from build123d import *

# Parameters (mm, degrees)
SKETCH_1_R                      = 21
EXTRUDE_1_DEPTH                 = 1.5
SKETCH_2_R                      = 21
SKETCH_2_R_2                    = 12
EXTRUDE_2_DEPTH                 = 2.2
SKETCH_7_R                      = 1.25
CUT_EXTRUDE_5_DEPTH             = 30.92808046
SKETCH_8_W                      = 14.034551426
SKETCH_8_H                      = 10.5
CUT_EXTRUDE_6_DEPTH             = 30.92808046
SKETCH_9_W                      = 17.42220177
SKETCH_9_H                      = 10.5
CUT_EXTRUDE_7_DEPTH             = 30.92808046
MOVE_BODY_5_ANGLE               = 45
MOVE_BODY_6_ANGLE               = 5
SKETCH_15_R                     = 0.55
SKETCH_15_R_2                   = 0.5
CUT_EXTRUDE_9_DEPTH             = 30.92808046
MOVE_BODY_7_ANGLE               = 49.5
SKETCH_16_R                     = 1.35
CUT_EXTRUDE_10_DEPTH            = 1.5
SKETCH_17_R                     = 2.5
CUT_EXTRUDE_11_DEPTH            = 2.2
SKETCH_23_R                     = 2
CUT_EXTRUDE_17_DEPTH            = 30.92808046
CUT_EXTRUDE_18_DEPTH            = 30.779858965
CUT_EXTRUDE_18_DEPTH_BACK       = 30.779858965
SKETCH_24_R                     = 1.6
CUT_EXTRUDE_25_DEPTH            = 30.92808046
SKETCH_42_R                     = 3
CUT_EXTRUDE_26_DEPTH            = 1
HOLE_WIZARD_3_100_1_D           = 3.048
HOLE_WIZARD_3_100_1_CSINK_D     = 5.0546
HOLE_WIZARD_3_100_1_CSINK_ANGLE = 100
CUT_EXTRUDE_27_DEPTH            = 30.92808046


with BuildPart() as part:
    # 草图1 → 凸台-拉伸1 (new body)
    with BuildSketch(Plane(origin=(0, 0, 0), x_dir=(1, 0, 0), z_dir=(0, 1, 0))):
        with Locations(Location((0, 0, 0), (0, 0, 270))):
            Circle(SKETCH_1_R)
    extrude(amount=EXTRUDE_1_DEPTH)

    # 草图2 → 凸台-拉伸2 (add)
    with BuildSketch(Plane(origin=(0, 1.5, 0), x_dir=(1, 0, 0), z_dir=(0, 1, 0))):
        with Locations(Location((0, 0, 0), (0, 0, 270))):
            Circle(SKETCH_2_R)
        with Locations(Location((0, 0, 0), (0, 0, 270))):
            Circle(SKETCH_2_R_2, mode=Mode.SUBTRACT)
    extrude(amount=EXTRUDE_2_DEPTH)

    # 草图7 → 切除-拉伸5 (cut, through all)
    with BuildSketch(Plane.XZ):
        with Locations(Location((-5.51, 9.05, 0), (0, 0, 270))):
            Circle(SKETCH_7_R)
        with Locations(Location((5.51, 9.05, 0), (0, 0, 270))):
            Circle(SKETCH_7_R)
        with Locations(Location((-5.51, -9.05, 0), (0, 0, 270))):
            Circle(SKETCH_7_R)
        with Locations(Location((5.51, -9.05, 0), (0, 0, 270))):
            Circle(SKETCH_7_R)
    extrude(amount=-CUT_EXTRUDE_5_DEPTH, mode=Mode.SUBTRACT)

    # 草图8 → 切除-拉伸6 (cut, through all)
    with BuildSketch(Plane.XZ):
        Rectangle(SKETCH_8_W, SKETCH_8_H)
    extrude(amount=-CUT_EXTRUDE_6_DEPTH, mode=Mode.SUBTRACT)

    # 草图9 → 切除-拉伸7 (cut, through all)
    with BuildSketch(Plane.XZ):
        with Locations((15.728376598, 0)):
            Rectangle(SKETCH_9_W, SKETCH_9_H)
    extrude(amount=-CUT_EXTRUDE_7_DEPTH, mode=Mode.SUBTRACT)


with BuildPart() as part_1:
    # Move Body 5: moved
    add(part.part.rotate(Axis((0, 0, 0), (0, 1, 0)), MOVE_BODY_5_ANGLE))


with BuildPart() as part_2:
    # Move Body 6: moved
    add(part_1.part.rotate(Axis((0, 0, 0), (0, 1, 0)), MOVE_BODY_6_ANGLE))

    # 草图15 → 切除-拉伸9 (cut, through all)
    with BuildSketch(Plane.XZ):
        with Locations(Location((-10.9, 10.9, 0), (0, 0, 270))):
            Circle(SKETCH_15_R)
        with Locations(Location((10.9, 10.9, 0), (0, 0, 270))):
            Circle(SKETCH_15_R_2)
        with Locations(Location((-10.9, -10.9, 0), (0, 0, 270))):
            Circle(SKETCH_15_R_2)
    extrude(amount=-CUT_EXTRUDE_9_DEPTH, mode=Mode.SUBTRACT)


with BuildPart() as part_3:
    # Move Body 7: moved
    add(part_2.part.rotate(Axis((0, 0, 0), (0, -1, 0)), MOVE_BODY_7_ANGLE))

    # 草图16 → 切除-拉伸10 (cut)
    with BuildSketch(Plane.XZ):
        with Locations(Location((-5.51, 9.05, 0), (0, 0, 270))):
            Circle(SKETCH_16_R)
        with Locations(Location((5.51, 9.05, 0), (0, 0, 270))):
            Circle(SKETCH_16_R)
        with Locations(Location((-5.51, -9.05, 0), (0, 0, 270))):
            Circle(SKETCH_16_R)
        with Locations(Location((5.51, -9.05, 0), (0, 0, 270))):
            Circle(SKETCH_16_R)
    extrude(amount=-CUT_EXTRUDE_10_DEPTH, mode=Mode.SUBTRACT)

    # 草图17 → 切除-拉伸11 (cut)
    with BuildSketch(Plane(origin=(0, 3.7, 0), x_dir=(1, 0, 0), z_dir=(0, 1, 0))):
        with Locations((-5.51, 9.05)):
            Circle(SKETCH_17_R)
        with Locations((5.51, 9.05)):
            Circle(SKETCH_17_R)
        with Locations((-5.51, -9.05)):
            Circle(SKETCH_17_R)
        with Locations((5.51, -9.05)):
            Circle(SKETCH_17_R)
    extrude(amount=-CUT_EXTRUDE_11_DEPTH, mode=Mode.SUBTRACT)

    # 草图23 → 切除-拉伸17 (cut, through all)
    with BuildSketch(Plane(origin=(0, 3.7, 0), x_dir=(1, 0, 0), z_dir=(0, 1, 0))):
        with Locations(Location((0, 16, 0), (0, 0, 270))):
            Circle(SKETCH_23_R)
        with Locations(Location((-16, 0, 0), (0, 0, 270))):
            Circle(SKETCH_23_R)
        with Locations(Location((0, -16, 0), (0, 0, 270))):
            Circle(SKETCH_23_R)
    extrude(amount=-CUT_EXTRUDE_17_DEPTH, mode=Mode.SUBTRACT)

    # 草图24 → 切除-拉伸18 (cut, two sides: drawn at the far end of the back side and taken through both)
    with BuildSketch(Plane(origin=(0, 1.5, 0), x_dir=(1, 0, 0), z_dir=(0, 1, 0)).offset(-CUT_EXTRUDE_18_DEPTH_BACK)):
        with Locations(Location((-5.51, 9.05, 0), (0, 0, 270))):
            Circle(SKETCH_24_R)
        with Locations(Location((5.51, 9.05, 0), (0, 0, 270))):
            Circle(SKETCH_24_R)
        with Locations(Location((-5.51, -9.05, 0), (0, 0, 270))):
            Circle(SKETCH_24_R)
        with Locations(Location((5.51, -9.05, 0), (0, 0, 270))):
            Circle(SKETCH_24_R)
    extrude(amount=CUT_EXTRUDE_18_DEPTH + CUT_EXTRUDE_18_DEPTH_BACK, mode=Mode.SUBTRACT)

    # 草图37 → 切除-拉伸25 (cut, through all)
    with BuildSketch(Plane.XZ):
        with BuildLine():
            Line((24.72756624, 20.266700409), (14.622140931, 20.266700409))
            Line((14.622140931, 20.266700409), (14.622140931, 15.072922563))
            ThreePointArc((14.622140931, 15.072922563), (18.200516902, 10.47574267), (20.378202654, 5.072362031))
            Line((20.378202654, 5.072362031), (14.622140931, 5.122594421))
            Line((14.622140931, 5.122594421), (14.622140931, -5.377805402))
            Line((14.622140931, -5.377805402), (20.286574032, -5.427238161))
            ThreePointArc((20.286574032, -5.427238161), (18.108406942, -10.634171243), (14.622140931, -15.072922563))
            Line((14.622140931, -15.072922563), (14.622140931, -20.266073881))
            Line((14.622140931, -20.266073881), (24.72756624, -20.266073881))
            Line((24.72756624, -20.266073881), (24.72756624, 20.266700409))
        make_face()
        with BuildLine():
            ThreePointArc((20.378202654, 5.072362031), (18.200516902, 10.47574267), (14.622140931, 15.072922563))
            Line((14.622140931, 15.072922563), (14.622140931, 5.122594421))
            Line((14.622140931, 5.122594421), (20.378202654, 5.072362031))
        make_face()
        with BuildLine():
            Line((14.622140931, -5.377805402), (14.622140931, -15.072922563))
            ThreePointArc((14.622140931, -15.072922563), (18.108406942, -10.634171243), (20.286574032, -5.427238161))
            Line((20.286574032, -5.427238161), (14.622140931, -5.377805402))
        make_face()
    extrude(amount=-CUT_EXTRUDE_25_DEPTH, mode=Mode.SUBTRACT)

    # 草图42 → 切除-拉伸26 (cut)
    with BuildSketch(Plane(origin=(0, 0, 0), x_dir=(-1, 0, 0), z_dir=(0, -1, 0))):
        with Locations(Location((-10.6, -10.6, 0), (0, 0, 90))):
            Circle(SKETCH_42_R)
        with Locations(Location((-10.6, 10.6, 0), (0, 0, 90))):
            Circle(SKETCH_42_R)
    extrude(amount=-CUT_EXTRUDE_26_DEPTH, mode=Mode.SUBTRACT)

    # #3 平头机械螺钉的锥形沉头孔 (100)1 (through all)
    with Locations(Plane(origin=(0, 0, 0), x_dir=(-1, 0, 0), z_dir=(0, -1, 0))):
        with Locations((10.6, -10.6), (-10.6, -10.6), (10.6, 10.6), (-10.6, 10.6)):
            CounterSinkHole(HOLE_WIZARD_3_100_1_D / 2, HOLE_WIZARD_3_100_1_CSINK_D / 2, counter_sink_angle=HOLE_WIZARD_3_100_1_CSINK_ANGLE)

    # 草图45 → 切除-拉伸27 (cut, through all)
    with BuildSketch(Plane(origin=(0, 3.7, 0), x_dir=(1, 0, 0), z_dir=(0, 1, 0))):
        with BuildLine():
            Line((-33, 4.25), (-14, 4.25))
            ThreePointArc((-14, 4.25), (-9.75, 0), (-14, -4.25))
            Line((-14, -4.25), (-33, -4.25))
            ThreePointArc((-33, -4.25), (-37.25, 0), (-33, 4.25))
        make_face()
        with BuildLine():
            Line((4.25, 33), (4.25, 14))
            ThreePointArc((4.25, 14), (0, 9.75), (-4.25, 14))
            Line((-4.25, 14), (-4.25, 33))
            ThreePointArc((-4.25, 33), (0, 37.25), (4.25, 33))
        make_face()
        with BuildLine():
            Line((-4.25, -33), (-4.25, -14))
            ThreePointArc((-4.25, -14), (0, -9.75), (4.25, -14))
            Line((4.25, -14), (4.25, -33))
            ThreePointArc((4.25, -33), (0, -37.25), (-4.25, -33))
        make_face()
    extrude(amount=-CUT_EXTRUDE_27_DEPTH, mode=Mode.SUBTRACT)


solid = part_3.part
Geometry check sheet. Reference: the model listing, model coordinates, mm. A direction names the side the tool comes from. Give positions to 0.01 mm unless a question says otherwise; leave off trailing zeros. Loops run counter-clockwise (first coordinate to the right, second up) from the corner with the lowest first, then second, coordinate; pieces in that order, holes last.
(1) Section check A-A on x = 0. Record the cut outline in (y, z).
From the geometry:
outline: (0, -9.75) - (1.5, -9.75) - (1.5, -5.25) - (0, -5.25) - close; (0, 5.25) - (1.5, 5.25) - (1.5, 9.75) - (0, 9.75) - close
(2) Section check C-C on x = 5.51. Record the cut outline in (y, z), then the cut area to 3 significant figures.
From the geometry:
outline: (0, -20.26) - (3.7, -20.26) - (3.7, -11.55) - (1.5, -11.55) - (1.5, -10.65) - (0, -10.65) - close; (0, -7.45) - (1.5, -7.45) - (1.5, -5.3) - (0, -5.3) - close; (0, 5.2) - (1.5, 5.2) - (1.5, 7.45) - (0, 7.45) - close; (0, 10.65) - (1.5, 10.65) - (1.5, 11.55) - (3.7, 11.55) - (3.7, 20.26) - (0, 20.26) - close
area: 73.8 mm2
(3) Section check B-B on z = -16. Record the cut outline in (x, y).
From the geometry:
outline: (-13.6, 0) - (-4.25, 0) - (-4.25, 3.7) - (-13.6, 3.7) - close; (4.25, 0) - (13.6, 0) - (13.6, 3.7) - (4.25, 3.7) - close
(4) Thickness scan on L1, parallel to Z at x = -5.51, y = 1.15; L2, parallel to Z at x = 5.51, y = 1.2; L3, parallel to Z at x = -16, y = 2.5. Record the ranges inside material, lowest first.
From the geometry:
L1: z = -20.26 to -10.65, -7.45 to -5.2, 5.3 to 7.45, 10.65 to 20.26
L2: z = -20.26 to -10.65, -7.45 to -5.3, 5.2 to 7.45, 10.65 to 20.26
L3: z = -13.6 to -4.25, 4.25 to 13.6
(5) Section check D-D on y = 3.2. Count the separate pieces of the cut face and the enclosed holes in it, then the cut area to 3 significant figures.
From the geometry:
separate pieces: 4
enclosed holes: 4
area: 498 mm2
(6) Depth check by flat-ended pin: pin 1 Ø1 at (x, y) = (-16, 2) entering from +Z; pin 2 Ø1.5 at (x, y) = (-6, 3) entering from +Z; pin 3 Ø1.8 at (x, z) = (10.5, -9) entering from -Y; pin 4 Ø2.5 at (x, z) = (-10.6, 10.6) entering from +Y. Enter the tip coordinate at first touch or a pass-through.
From the geometry:
pin 1: stops at z = 14.17
pin 2: stops at z = 20.33
pin 3: stops at y = 1
pin 4: passes through
(7) Set-up check for faces 1 (the flat face through (9, 1, 9)), 2 (the flat face through (4.25, 2, 17)), 3 (the flat face through (-8, 1.5, 0)): record each of +Z, -Z, +X, -X, +Y, -Y from which the full face is reachable in a straight line by a thin tool's end or side.
From the geometry:
face 1: -Y
face 2: +Z, +Y, -Y
face 3: +Y
(8) Release check for a two-part mould opening along X. For faces 4 (the flat face through (10, 3.7, -13)), 5 (the cylindrical face through (-12.123, 2.291, -10.667)), 6 (the cylindrical face through (9.75, 1.82, 18.6)) record: released by +X, released by -X, zero draft, split by the parting line, or undercut.
From the geometry:
face 4: zero draft
face 5: undercut
face 6: released by +X
